Build history of the part. All positions in model axes, mm. A direction names the side the tool comes from. Coordinates: 2 decimals unless noted, no trailing zeros. Order: outer loops, then holes, each group sorted by start corner. A loop starts at its lowest first (then second) coordinate and runs counter-clockwise, first axis right, second up. Notation, with made-up numbers: (51.25, 10.25) - (89.25, 10.25) arc R31 cw to (89.25, 47.25) - close; hole circle Ø9 at (58, 89). An arc over 180 degrees is marked (long way). Write each question's results on one line, items separated by ' | '.
from build123d import *

# Parameters (mm, degrees)
BOSS_EXTRUDE1_DEPTH      = 7.5
BOSS_EXTRUDE1_DEPTH_BACK = 7.5
SKETCH1_R                = 10
SKETCH1_R_2              = 3
BOSS_EXTRUDE2_DEPTH      = 12.5
BOSS_EXTRUDE2_DEPTH_BACK = 12.5
SKETCH1_2_R              = 10
SKETCH1_2_R_2            = 3


with BuildPart() as part:
    # Sketch1 → Boss-Extrude1 (new, two sides: drawn at the far end of the back side and taken through both)
    # profile 1 of 2: a face of its own
    with BuildSketch(Plane.XY.offset(-BOSS_EXTRUDE1_DEPTH_BACK)):
        Circle(SKETCH1_R)
        Circle(SKETCH1_R_2, mode=Mode.SUBTRACT)
    # profile 2 of 2: a face of its own
    with BuildSketch(Plane.XY.offset(-BOSS_EXTRUDE1_DEPTH_BACK)):
        Circle(SKETCH1_R_2)
    extrude(amount=BOSS_EXTRUDE1_DEPTH + BOSS_EXTRUDE1_DEPTH_BACK)

    # Sketch1_2 → Boss-Extrude2 (add, two sides: drawn at the far end of the back side and taken through both)
    with BuildSketch(Plane.XY.offset(-BOSS_EXTRUDE2_DEPTH_BACK)):
        Circle(SKETCH1_2_R)
        Circle(SKETCH1_2_R_2, mode=Mode.SUBTRACT)
    extrude(amount=BOSS_EXTRUDE2_DEPTH + BOSS_EXTRUDE2_DEPTH_BACK)


solid = part.part
1. Band-saw the part on C-C on z = 10.5. Give the cut face in (x, y).
Solved:
outline: circle Ø20 at (0, 0); hole circle Ø6 at (0, 0)
2. Tool access for faces 1 (the face through (2.1, 2.4, -12.5)), 2 (the face through (0, 0, 7.5)), 3 (the face through (-3, 0, -10)): list every direction of +Z, -Z, +X, -X, +Y, -Y with a clear straight run to the whole face (end or side of a thin tool).
Solved:
face 1: -Z, +X, -X, +Y, -Y | face 2: +Z | face 3: -Z
3. Two-plate mould, pull along X, no slides. Class faces 4 (the face through (2.1, 2.4, 12.5)), 5 (the face through (-3, 0, 10)), 6 (the face through (-2.17, -9.76, -0.18)): +X half, -X half, draft (parallel to the pull), parting line (faces both ways), or undercut.
Solved:
face 4: draft | face 5: undercut | face 6: parting line
4. Probe line 1 (Y direction, x = 0, z = -10.6); line 2 (Z direction, x = 0.5, y = 2.75); line 3 (X direction, y = -4.5, z = 11.25). List the from-to ranges inside material, lowest first.
Solved:
line 1: y = -10 to -3, 3 to 10 | line 2: z = -7.5 to 7.5 | line 3: x = -8.93 to 8.93
5. Band-saw the part on D-D on z = 5.75. Give the cut face in (x, y), then the cut area to 3 significant figures.
Solved:
outline: circle Ø20 at (0, 0) | area: 314 mm2
6. Band-saw the part on A-A on x = 0. Give the cut face in (y, z), then the cut area to 3 significant figures.
Solved:
outline: (-10, -12.5) - (-3, -12.5) - (-3, -7.5) - (3, -7.5) - (3, -12.5) - (10, -12.5) - (10, 12.5) - (3, 12.5) - (3, 7.5) - (-3, 7.5) - (-3, 12.5) - (-10, 12.5) - close | area: 440 mm2
7. Drop flat-ended pins along their axis: pin 1 Ø4 at (x, z) = (-5.5, -8) entering from -Y; pin 2 Ø3.5 at (x, y) = (0, 0) entering from +Z; pin 3 Ø1.5 at (y, z) = (1.5, -5) entering from +X. Give the stop position or say it passes through.
Solved:
pin 1: stops at y = -9.37 | pin 2: stops at z = 7.5 | pin 3: stops at x = 9.97
